from build123d import *

# Parameters (mm, degrees)
PAD_DEPTH       = 10
SKETCH001_W     = 3
SKETCH001_H     = 8
POCKET_DEPTH    = 22
POCKET001_DEPTH = 5
SKETCH003_R     = 1.7
POCKET002_DEPTH = 5
PAD001_DEPTH    = 35
SKETCH005_W     = 9
SKETCH005_H     = 3
POCKET003_DEPTH = 7
SKETCH009_R     = 1.146705
SKETCH009_R_2   = 1.359748
POCKET005_DEPTH = 10.501
SKETCH010_R     = 1.3
POCKET006_DEPTH = 5


with BuildPart() as part:
    # Sketch → Pad (new body)
    with BuildSketch(Plane.XY):
        Polygon((12.5, 29), (22.5, 29), (22.5, 4), (35, 4), (35, 0), (0, 0), (0, 4), (12.5, 4), align=None)
    extrude(amount=PAD_DEPTH)

    # Sketch001 → Pocket (cut)
    with BuildSketch(Plane(origin=(0, 29, 0), x_dir=(-1, 0, 0), z_dir=(0, 1, 0))):
        with Locations((-17.5, 5)):
            Rectangle(SKETCH001_W, SKETCH001_H)
    extrude(amount=-POCKET_DEPTH, mode=Mode.SUBTRACT)

    # Sketch002 → Pocket001 (cut)
    with BuildSketch(Plane(origin=(12.5, 0, 0), x_dir=(0, -1, 0), z_dir=(-1, 0, 0))):
        with BuildLine():
            ThreePointArc((-29, 1), (-25, 5), (-29, 9))
            Line((-29, 9), (-29, 1))
        make_face()
    extrude(amount=-POCKET001_DEPTH, mode=Mode.SUBTRACT)

    # Sketch003 → Pocket002 (cut)
    with BuildSketch(Plane.YZ.offset(22.5)):
        with Locations((26.5, 5)):
            Circle(SKETCH003_R)
    extrude(amount=-POCKET002_DEPTH, mode=Mode.SUBTRACT)

    # Sketch004 → Pad001 (new body)
    with BuildSketch(Plane(origin=(0, 0, 0), x_dir=(0, -1, 0), z_dir=(-1, 0, 0))):
        Polygon((0, 0), (6.5, 0), (6.5, 10), (3.5, 10), (3.5, 3), (0, 3), align=None)
    extrude(amount=-PAD001_DEPTH)

    # Sketch005 → Pocket003 (cut)
    with BuildSketch(Plane.XY.offset(10)):
        with Locations((17.5, -5)):
            Rectangle(SKETCH005_W, SKETCH005_H)
    extrude(amount=-POCKET003_DEPTH, mode=Mode.SUBTRACT)

    # Sketch009 → Pocket005 (cut, through all)
    with BuildSketch(Plane(origin=(0, 4, 0), x_dir=(-1, 0, 0), z_dir=(0, 1, 0))):
        with Locations((-28.59808, 5.511153)):
            Circle(SKETCH009_R)
        with Locations((-5.681909, 5.536989)):
            Circle(SKETCH009_R_2)
    extrude(amount=-POCKET005_DEPTH, mode=Mode.SUBTRACT)

    # Sketch010 → Pocket006 (cut)
    with BuildSketch(Plane.YZ.offset(22.5)):
        with Locations((20.5, 5)):
            Circle(SKETCH010_R)
    extrude(amount=-POCKET006_DEPTH, mode=Mode.SUBTRACT)


solid = part.part
Model file for the job. Use its own axes, mm. A direction names the side the tool comes from. Give positions to 0.01 mm unless a question says otherwise; leave off trailing zeros. Write each loop counter-clockwise with the first axis right and the second up, starting at its lowest first coordinate (ties: lowest second). Pieces come first, ordered by that corner, then holes. Notation, with made-up numbers: (46, -39.5) - (74, -39.5) arc R8 cw to (74, -33.5) - close; hole circle Ø2 at (16, -30). An arc over 180 degrees is marked (long way). Answer as CSV lines item,"result".
1. Band-saw the part on A-A (y = 10). Write the cut outline in (x, z), and give its area (3 significant figures).
Responses:
outline,"(12.5, 0) - (22.5, 0) - (22.5, 10) - (12.5, 10) - close; hole (16, 1) - (19, 1) - (19, 9) - (16, 9) - close"
area,"76.0 mm2"
2. Drill centre lines: L1, parallel to X at y = 22, z = 4.5; L2, parallel to Y at x = 8, z = 6.75; L3, parallel to X at y = -4, z = 9.25. Where is each one in solid material? Low to high. Write a range as [from, to].
Responses:
L1,"x = [12.5, 16], [19, 22.5]"
L2,"y = [-6.5, -3.5], [0, 4]"
L3,"x = [0, 13], [22, 35]"
3. Band-saw the part on B-B (x = 15). Write the cut outline in (y, z), and give its area (3 significant figures).
Responses:
outline,"(-6.5, 0) - (29, 0) - (29, 1) arc R4 cw to (29, 9) - (29, 10) - (0, 10) - (0, 3) - (-6.5, 3) - close"
area,"284 mm2"
4. Band-saw the part on C-C (y = 26.5). Write the cut outline in (x, z).
Responses:
outline,"(12.5, 0) - (22.5, 0) - (22.5, 3.3) - (19, 3.3) - (19, 1) - (16, 1) - (16, 1.88) - (12.5, 1.88) - close; (12.5, 8.12) - (16, 8.12) - (16, 9) - (19, 9) - (19, 6.7) - (22.5, 6.7) - (22.5, 10) - (12.5, 10) - close"
5. Band-saw the part on D-D (z = 5). Count the separate pieces of the cut face and the enclosed holes in it, and give its area (3 significant figures).
Responses:
separate pieces,"9"
enclosed holes,"0"
area,"335 mm2"
6. Two-plate mould, pull along Z, no slides. Class faces 5 (the face through (12.5, 16, 5)), 6 (the face through (17, 8, 0)), 7 (the face through (19, 18, 5)): +Z half, -Z half, draft (parallel to the pull), parting line (faces both ways), or undercut.
Responses:
face 5,"draft"
face 6,"-Z half"
face 7,"undercut"
7. Pin check, flat tips, straight feed: pin 1 (2 mm diameter, centred on x = 5.68, z = 5.54, fed in from +Y); pin 2 (1 mm diameter, centred on x = 26, z = 9, fed in from +Y); pin 3 (1.6 mm diameter, centred on y = 20.5, z = 5, fed in from -X); pin 4 (4 mm diameter, centred on y = 26.5, z = 5, fed in from +X). Stop position of each tip, or through.
Responses:
pin 1,"passes through"
pin 2,"stops at y = 4"
pin 3,"stops at x = 12.5"
pin 4,"stops at x = 22.5"
8. 3-axis set-ups, long thin cutter, end or side, ignore diameter. For faces 1 (the face through (16, 16, 5)), 2 (the face through (14, 25, 5)), 3 (the face through (22, -5, 7)), 4 (the face through (6, 4, 4)): which of +Z, -Z, +X, -X, +Y, -Y reach the whole face in a straight line?
Responses:
face 1,"+Y"
face 2,"-X, +Y"
face 3,"+Z, -Y"
face 4,"+Z, -Z, -X, +Y"
